Source: CAD feature listing. Evaluate the final solid. Frame: model axes, mm. A direction names the side the tool comes from. Give positions to 0.01 mm unless a question says otherwise; leave off trailing zeros. Write item = value, one per line.
from build123d import *

# Parameters (mm, degrees)
BOSS_EXTRUDE1_DEPTH = 5.842
SKETCH3_W           = 38.1
SKETCH3_H           = 50.8
SKETCH3_W_2         = 3.048
CUT_EXTRUDE1_DEPTH  = 243.64734842


with BuildPart() as part:
    # Sketch2 → Boss-Extrude1 (new body)
    with BuildSketch(Plane.XY):
        with BuildLine():
            Line((132.489119036, 39.6875), (0, 39.6875))
            Line((0, 39.6875), (0, 203.2))
            add(Edge.make_bspline(
                [(0, 203.2), (17.235406981, 203.2), (50.061159208, 185.921315787), (85.218169736, 152.2019324), (115.206186784, 104.366247761), (132.489119036, 63.290972919), (132.489119036, 39.6875)],
                knots=[0, 0, 0, 0, 0.231795721, 0.463575912, 0.653721915, 1, 1, 1, 1], degree=3))
        make_face()
    extrude(amount=BOSS_EXTRUDE1_DEPTH)

    # Sketch3 → Cut-Extrude1 (cut, through all)
    with BuildSketch(Plane.XY.offset(5.842)):
        with Locations((19.05, 65.0875)):
            Rectangle(SKETCH3_W, SKETCH3_H)
        with Locations((1.524, 177.8)):
            Rectangle(SKETCH3_W_2, SKETCH3_H)
    extrude(amount=-CUT_EXTRUDE1_DEPTH, mode=Mode.SUBTRACT)

    # Mirror1: part across plane


with BuildPart() as part_1:
    add(part.part)
    add(part.part.mirror(Plane(origin=(0, 0, 0), x_dir=(0, 0, 1), z_dir=(1, 0, 0))))


solid = part_1.part
(1) Access query for faces 1 (the face through (-3.048, 177, 3)), 2 (the face through (1, 90.488, 3)), 3 (the face through (-86, 39.688, 3)). Directions: +Z, -Z, +X, -X, +Y, -Y. A direction counts if a zero-diameter tool reaches every point of the face in a straight line with its end or side. Return the directions, or none.
Values follow:
face_1 = +Z, -Z, +Y
face_2 = +Z, -Z, -Y
face_3 = +Z, -Z, +X, -X, -Y
(2) Pull-direction query (X, two-part tool) for faces 4 (the face through (38.1, 65, 3)), 5 (the face through (-2, 104, 0)), 6 (the face through (-38.1, 65, 3)); classes: pulls with the +X half, pulls with the -X half, needs draft (parallel to the pull), parting line crosses it, or undercut.
Values follow:
face_4 = undercut
face_5 = needs draft
face_6 = undercut
(3) Material intervals for line 1 (X direction, y = 78.5, z = 3.2); line 2 (X direction, y = 188, z = 0.8); line 3 (Y direction, x = 99.5, z = 5.3), sorted ascending.
Values follow:
line_1 = -124.62 to -38.1, 38.1 to 124.62
line_2 = -42.63 to -3.05, 3.05 to 42.63
line_3 = 39.69 to 128.87
(4) First-contact query: pin 1 (3 mm diameter, centred on y = 167.5, z = 3, fed in from +X); pin 2 (1.8 mm diameter, centred on x = -1, z = 2, fed in from -Y); pin 3 (4 mm diameter, centred on x = -30, y = 88, fed in from -Z); pin 4 (3 mm diameter, centred on y = 71.5, z = 4.5, fed in from +X). Flat tips, straight axial feed; report the tip coordinate or a pass-through.
Values follow:
pin_1 = 69.95
pin_2 = 90.49
pin_3 = through
pin_4 = 127.46
